Verification items for the finished model (mm, model axes). A direction names the side the tool comes from. Coordinates: 2 decimals unless noted, no trailing zeros. Order: outer loops, then holes, each group sorted by start corner. A loop starts at its lowest first (then second) coordinate and runs counter-clockwise, first axis right, second up.
Q1. Thickness scan on line 1 (Y direction, x = 10, z = 1.3); line 2 (X direction, y = 20, z = 12.5); line 3 (Z direction, x = 28.5, y = 18). Record the ranges inside material, lowest first.
Q2. Depth check by flat-ended pin: P1, Ø12, axis at x = 15, y = 34.5, coming from the +Z side; P2, Ø6.5, axis at y = 20, z = 9, coming from the -X side. Enter the tip coordinate at first touch or a pass-through.
Q3. Draft check along X on faces 4 (the cylindrical face through (39.1, 0.86, 2.54)), 5 (the flat face through (27.361, 35.896, 2.535)), 6 (the flat face through (20, 20, 0)). Enter one of: pulls with the +X half, pulls with the -X half, needs draft (parallel to the pull), parting line crosses it, or undercut.
Q4. Set-up check for faces 1 (the flat face through (20, 20, 5)), 2 (the flat face through (27.336, 4.128, 2.535)), 3 (the cylindrical face through (4.9, 19.9, 15.5)): record each of +Z, -Z, +X, -X, +Y, -Y from which the full face is reachable in a straight line by a thin tool's end or side.
Q5. Cross-section at B-B, the plane y = 20. Record the boundary of the cut face in (x, z).
Q6. Cross-section at D-D, the plane z = 9.5. Record the boundary of the cut face in (x, y).
Q7. Cross-section at A-A, the plane x = 12. Record the boundary of the cut face in (y, z), and give its area (3 significant figures).
Q8. Cross-section at C-C, the plane z = 2.25. Record the boundary of the cut face in (x, y), and give its area (3 significant figures).
from build123d import *

# Parameters (mm, degrees)
SKETCH1_W              = 40
SKETCH1_H              = 40
BOSS_EXTRUDE1_DEPTH    = 5
CUT_EXTRUDE1_DEPTH     = 57.789083458
SKETCH3_R              = 2.5
BOSS_EXTRUDE2_DEPTH    = 10
FILLET1_R              = 3
LPATTERN1_COUNT        = 2
LPATTERN1_PITCH        = 30
FILLET1_OF_LPATTERN1_R = 3
FILLET2_R              = 3


with BuildPart() as part:
    # Sketch1 → Boss-Extrude1 (new body)
    with BuildSketch(Plane.XY):
        with Locations((20, 20)):
            Rectangle(SKETCH1_W, SKETCH1_H)
    extrude(amount=BOSS_EXTRUDE1_DEPTH)

    # Sketch2 → Cut-Extrude1 (cut, through all)
    with BuildSketch(Plane.XY.offset(5)):
        with BuildLine():
            Line((8.232233047, 36.767766953), (6.464466094, 35))
            Line((6.464466094, 35), (8.232233047, 33.232233047))
            ThreePointArc((8.232233047, 33.232233047), (12.5, 35), (8.232233047, 36.767766953))
        make_face()
        with BuildLine():
            Line((26.464466094, 35), (28.232233047, 33.232233047))
            ThreePointArc((28.232233047, 33.232233047), (32.5, 35), (28.232233047, 36.767766953))
            Line((28.232233047, 36.767766953), (26.464466094, 35))
        make_face()
        with BuildLine():
            Line((26.464466094, 5), (28.232233047, 3.232233047))
            ThreePointArc((28.232233047, 3.232233047), (32.5, 5), (28.232233047, 6.767766953))
            Line((28.232233047, 6.767766953), (26.464466094, 5))
        make_face()
        with BuildLine():
            Line((6.464466094, 5), (8.232233047, 3.232233047))
            ThreePointArc((8.232233047, 3.232233047), (12.5, 5), (8.232233047, 6.767766953))
            Line((8.232233047, 6.767766953), (6.464466094, 5))
        make_face()
    extrude(amount=-CUT_EXTRUDE1_DEPTH, mode=Mode.SUBTRACT)

    # Sketch3 → Boss-Extrude2 (add)
    with BuildSketch(Plane.ZY):
        with BuildLine():
            Line((12.355222683, 25.567089073), (5, 30))
            Line((5, 30), (5, 10))
            Line((5, 10), (12.355222683, 14.432910927))
            ThreePointArc((12.355222683, 14.432910927), (15.5, 20), (12.355222683, 25.567089073))
        make_face()
        with Locations((9, 20)):
            Circle(SKETCH3_R, mode=Mode.SUBTRACT)
    boss_extrude2 = extrude(amount=-BOSS_EXTRUDE2_DEPTH)

    # Fillet1
    fillet1_edges = [part.edges().sort_by_distance(p)[0] for p in [
        (5, 10, 5),
        (5, 30, 5),
    ]]
    fillet(fillet1_edges, radius=FILLET1_R)

    # LPattern1: Boss-Extrude2 ×2
    with Locations(*[(i * LPATTERN1_PITCH, 0, 0) for i in range(1, LPATTERN1_COUNT)]):
        add(boss_extrude2)

    # Fillet1 of LPattern1
    fillet1_of_lpattern1_edges = [part.edges().sort_by_distance(p)[0] for p in [
        (35, 10, 5),
        (35, 30, 5),
    ]]
    fillet(fillet1_of_lpattern1_edges, radius=FILLET1_OF_LPATTERN1_R)

    # Fillet2
    fillet2_edges = [part.edges().sort_by_distance(p)[0] for p in [
        (0, 40, 2.5),
        (40, 40, 2.5),
        (40, 0, 2.5),
        (0, 0, 2.5),
    ]]
    fillet(fillet2_edges, radius=FILLET2_R)


solid = part.part
Check values:
1. line 1: y = 0 to 2.5, 7.5 to 32.5, 37.5 to 40
1. line 2: x = 0 to 10, 30 to 40
1. line 3: z = 0 to 5
2. P1: stops at z = 5.04
2. P2: stops at x = 0
3. face 4: pulls with the +X half
3. face 5: undercut
3. face 6: needs draft
4. face 1: +Z
4. face 2: +Z, -Z
4. face 3: +Z, +X, -X
5. outline: (0, 0) - (40, 0) - (40, 6.5) - (30, 6.5) - (30, 5) - (10, 5) - (10, 6.5) - (0, 6.5) - close; (0, 11.5) - (10, 11.5) - (10, 15.5) - (0, 15.5) - close; (30, 11.5) - (40, 11.5) - (40, 15.5) - (30, 15.5) - close
6. outline: (0, 12.71) - (10, 12.71) - (10, 17.55) - (0, 17.55) - close; (0, 22.45) - (10, 22.45) - (10, 27.29) - (0, 27.29) - close; (30, 12.71) - (40, 12.71) - (40, 17.55) - (30, 17.55) - close; (30, 22.45) - (40, 22.45) - (40, 27.29) - (30, 27.29) - close
7. outline: (0, 0) - (3.5, 0) - (3.5, 5) - (0, 5) - close; (6.5, 0) - (33.5, 0) - (33.5, 5) - (6.5, 5) - close; (36.5, 0) - (40, 0) - (40, 5) - (36.5, 5) - close
7. area: 170 mm2
8. outline: (0, 3) arc R3 ccw to (3, 0) - (37, 0) arc R3 ccw to (40, 3) - (40, 37) arc R3 ccw to (37, 40) - (3, 40) arc R3 ccw to (0, 37) - close; hole (6.46, 5) - (8.23, 3.23) arc R2.5 ccw (long way) to (8.23, 6.77) - close; hole (6.46, 35) - (8.23, 33.23) arc R2.5 ccw (long way) to (8.23, 36.77) - close; hole (26.46, 5) - (28.23, 3.23) arc R2.5 ccw (long way) to (28.23, 6.77) - close; hole (26.46, 35) - (28.23, 33.23) arc R2.5 ccw (long way) to (28.23, 36.77) - close
8. area: 1,510 mm2
